from build123d import *

# Parameters (mm, degrees)
SKETCH_1_W      = 365
SKETCH_1_H      = 228
EXTRUDE_1_DEPTH = 75
SKETCH_2_R      = 7.5
EXTRUDE_2_DEPTH = 15
FILLET_1_R      = 2


with BuildPart() as part:
    # 草图1 → 凸台-拉伸1 (new body)
    with BuildSketch(Plane(origin=(0, 0, 0), x_dir=(1, 0, 0), z_dir=(0, 1, 0))):
        Rectangle(SKETCH_1_W, SKETCH_1_H)
    extrude(amount=EXTRUDE_1_DEPTH)

    # 草图2 → 凸台-拉伸2 (add)
    with BuildSketch(Plane.ZY.offset(182.5)):
        with Locations(Location((-86, 37.5, 0), (0, 0, 180))):
            Circle(SKETCH_2_R)
        with Locations(Location((86, 37.5, 0), (0, 0, 180))):
            Circle(SKETCH_2_R)
    extrude(amount=EXTRUDE_2_DEPTH)

    # 圆角1
    fillet_1_edges = [part.edges().sort_by_distance(p)[0] for p in [
        (182.5, 75, 0),
        (0, 75, -114),
        (-182.5, 75, 0),
        (0, 0, -114),
        (182.5, 0, 0),
        (0, 0, 114),
        (-182.5, 0, 0),
        (-182.5, 37.5, -114),
        (182.5, 37.5, -114),
        (182.5, 37.5, 114),
        (-182.5, 37.5, 114),
        (0, 75, 114),
    ]]
    fillet(fillet_1_edges, radius=FILLET_1_R)


solid = part.part
Here's how the part is built. I have some questions about the finished solid (model axes, mm). A direction names the side the tool comes from. Give positions to 0.01 mm unless a question says otherwise; leave off trailing zeros. Write each loop counter-clockwise with the first axis right and the second up, starting at its lowest first coordinate (ties: lowest second). Pieces come first, ordered by that corner, then holes. Notation, with made-up numbers: (-5.75, 37) -> (13.25, 37) arc R9 cw to (13.25, 42) -> close; hole circle Ø9 at (24, 83). An arc over 180 degrees is marked (long way). Use one line per item in the form item = value. Start each with the question number.
1. Imagine slicing it at B-B on z = -40.5. List the corners of the cut face in (x, y) for me, plus the area to 3 significant figures.
2. If I drill on L1, parallel to X at y = 18, z = -52.5; L2, parallel to Y at x = -181, z = -33.5, over which ranges is the centre line in solid material (lowest first)?
3. Imagine slicing it at A-A on y = 9. List the corners of the cut face in (x, z) for me, plus the area to 3 significant figures.
4. Imagine slicing it at D-D on z = 86. List the corners of the cut face in (x, y) for me, plus the area to 3 significant figures.
5. On a 3-axis mill with a long thin cutter (end or side, diameter ignored), from which of +Z, -Z, +X, -X, +Y, -Y can I reach the whole of each face in a straight line? I mean faces 1 (the face through (-189.9, 44.82, 87.63)), 2 (the face through (-3, 75, -2)). Say none if no direction works.
6. Thinking about a two-plate mould opening in Z: for faces 3 (the face through (-3, 0, -2)), 4 (the face through (-3, 37, -114)), 5 (the face through (-189.9, 44.82, -84.37)), which applies, +Z half, -Z half, draft (parallel to the pull), parting line (faces both ways), or undercut?
7. Will this pin go through, and if not, where does the flat tip stop? pin 1 Ø4 at (y, z) = (53, 69.5) entering from -X.
8. Imagine slicing it at C-C on y = 37.5. List the corners of the cut face in (x, z) for me, plus the area to 3 significant figures.
Entries:
q1.outline = (-182.5, 2) arc R2 ccw to (-180.5, 0) -> (180.5, 0) arc R2 ccw to (182.5, 2) -> (182.5, 73) arc R2 ccw to (180.5, 75) -> (-180.5, 75) arc R2 ccw to (-182.5, 73) -> close
q1.area = 27,400 mm²
q2.L1 = -182.5 to 182.5
q2.L2 = 0.06 to 74.94
q3.outline = (-182.5, -112) arc R2 ccw to (-180.5, -114) -> (180.5, -114) arc R2 ccw to (182.5, -112) -> (182.5, 112) arc R2 ccw to (180.5, 114) -> (-180.5, 114) arc R2 ccw to (-182.5, 112) -> close
q3.area = 83,200 mm²
q4.outline = (-197.5, 30) -> (-182.5, 30) -> (-182.5, 2) arc R2 ccw to (-180.5, 0) -> (180.5, 0) arc R2 ccw to (182.5, 2) -> (182.5, 73) arc R2 ccw to (180.5, 75) -> (-180.5, 75) arc R2 ccw to (-182.5, 73) -> (-182.5, 45) -> (-197.5, 45) -> close
q4.area = 27,600 mm²
q5.face_1 = -X
q5.face_2 = +Z, -Z, +X, -X, +Y
q6.face_3 = draft
q6.face_4 = -Z half
q6.face_5 = undercut
q7.pin_1 = -182.5
q8.outline = (-197.5, -93.5) -> (-182.5, -93.5) -> (-182.5, -112) arc R2 ccw to (-180.5, -114) -> (180.5, -114) arc R2 ccw to (182.5, -112) -> (182.5, 112) arc R2 ccw to (180.5, 114) -> (-180.5, 114) arc R2 ccw to (-182.5, 112) -> (-182.5, 93.5) -> (-197.5, 93.5) -> (-197.5, 78.5) -> (-182.5, 78.5) -> (-182.5, -78.5) -> (-197.5, -78.5) -> close
q8.area = 83,700 mm²
